```python
from build123d import *

# Parameters (mm, degrees)
STOCK_DGT_START                               = 23.8125
STOCK_DGT_INSIDE_SWERVE_STRUCTURE_SM_2_R      = 28.175
STOCK_DGT_INSIDE_SWERVE_STRUCTURE_SM_2_R_2    = 2.2479
STOCK_DGT_INSIDE_SWERVE_STRUCTURE_SMALL_DEPTH = 4.7625
FILLET1_R                                     = 1.905


# Read off the part's stored shape, not the designer's step: Stock-DGT inside swerve structure Small Bearing-1
with BuildPart() as part:
    # Stock-DGT inside swerve structure Sm 2 → Stock-DGT inside swerve structure Small Bearing-1 (new body)
    with BuildSketch(Plane(origin=(0, 0, 0), x_dir=(1, 0, 0), z_dir=(0, 1, 0)).offset(STOCK_DGT_START)):
        Circle(STOCK_DGT_INSIDE_SWERVE_STRUCTURE_SM_2_R)
        with Locations((-14.933176064, -16.8275)):
            Circle(STOCK_DGT_INSIDE_SWERVE_STRUCTURE_SM_2_R_2, mode=Mode.SUBTRACT)
        with Locations((14.933176064, -16.8275)):
            Circle(STOCK_DGT_INSIDE_SWERVE_STRUCTURE_SM_2_R_2, mode=Mode.SUBTRACT)
        with Locations((-14.933176064, 16.8275)):
            Circle(STOCK_DGT_INSIDE_SWERVE_STRUCTURE_SM_2_R_2, mode=Mode.SUBTRACT)
        with BuildLine():
            ThreePointArc((11.1125, 13.879508051), (12.572358569, 12.572358569), (13.879508051, 11.1125))
            Line((13.879508051, 11.1125), (22.394471276, 11.1125))
            ThreePointArc((22.394471276, 11.1125), (25, 0), (22.394471276, -11.1125))
            Line((22.394471276, -11.1125), (13.879508051, -11.1125))
            ThreePointArc((13.879508051, -11.1125), (12.572358569, -12.572358569), (11.1125, -13.879508051))
            Line((11.1125, -13.879508051), (11.1125, -19.116031394))
            Line((11.1125, -19.116031394), (-11.1125, -19.116031394))
            Line((-11.1125, -19.116031394), (-11.1125, -11.33701763))
            ThreePointArc((-11.1125, -11.33701763), (-15.875, 0), (-11.1125, 11.33701763))
            Line((-11.1125, 11.33701763), (-11.1125, 19.116031394))
            Line((-11.1125, 19.116031394), (11.1125, 19.116031394))
            Line((11.1125, 19.116031394), (11.1125, 13.879508051))
        make_face(mode=Mode.SUBTRACT)
        with Locations((14.933176064, 16.8275)):
            Circle(STOCK_DGT_INSIDE_SWERVE_STRUCTURE_SM_2_R_2, mode=Mode.SUBTRACT)
    extrude(amount=STOCK_DGT_INSIDE_SWERVE_STRUCTURE_SMALL_DEPTH)

    # Fillet1
    fillet1_edges = [part.edges().sort_by_distance(p)[0] for p in [
        (22.394471276, 26.19375, 11.1125),
        (22.394471276, 26.19375, -11.1125),
        (11.1125, 26.19375, 13.879508051),
        (11.1125, 26.19375, -13.879508051),
        (13.879508051, 26.19375, -11.1125),
        (13.879508051, 26.19375, 11.1125),
        (-11.1125, 26.19375, -11.33701763),
        (-11.1125, 26.19375, 11.33701763),
        (11.1125, 26.19375, -19.116031394),
        (-11.1125, 26.19375, 19.116031394),
        (11.1125, 26.19375, 19.116031394),
        (-11.1125, 26.19375, -19.116031394),
    ]]
    fillet(fillet1_edges, radius=FILLET1_R)


solid = part.part
```
Check sheet for the modelled part. Datum: model origin and axes. Units: mm. Round coordinates to 2 decimals unless told otherwise and drop trailing zeros. Loops run counter-clockwise (first coordinate to the right, second up) from the corner with the lowest first, then second, coordinate; pieces in that order, holes last. Notation, with made-up numbers: (-7, 47) -> (19, 47) arc R25 ccw to (19, 75) -> close; hole circle Ø1 at (-23, -37.75). An arc over 180 degrees is marked (long way). Answer in a Markdown table with one row per item.
Q1. Go/stop test with flat-tipped pins: P1, Ø1.4, axis at x = 18, y = 27, coming from the +Z side; P2, Ø4, axis at x = -14.93, z = 16.83, coming from the +Y side; P3, Ø2.5, axis at y = 27, z = -16, coming from the -X side; P4, Ø2, axis at y = 26.5, z = 16, coming from the -X side. Record where each tip stops, or that it passes through.
Data:
| item | result |
|---|---|
| P1 | stops at z = 22.24 |
| P2 | passes through |
| P3 | stops at x = -24.01 |
| P4 | stops at x = -23.85 |
Q2. Sectioned sample at A-A on x = 0. Enter the section's corners in (y, z) (1 decimal).
Data:
| item | result |
|---|---|
| outline | (23.8, -28.2) -> (28.6, -28.2) -> (28.6, -19.1) -> (23.8, -19.1) -> close; (23.8, 19.1) -> (28.6, 19.1) -> (28.6, 28.2) -> (23.8, 28.2) -> close |
Q3. Thickness scan on L1, parallel to Z at x = 0.5, y = 26.5; L2, parallel to Z at x = 14, y = 24.9; L3, parallel to X at y = 27.4, z = 17.5. Record the ranges inside material, lowest first.
Data:
| item | result |
|---|---|
| L1 | z = -28.17 to -19.12, 19.12 to 28.17 |
| L2 | z = -24.45 to -18.87, -14.78 to -11.27, 11.27 to 14.78, 18.87 to 24.45 |
| L3 | x = -22.08 to -17.08, -12.79 to -11.09, 11.09 to 12.79, 17.08 to 22.08 |
Q4. Sectioned sample at C-C on z = -18. Enter the section's corners in (x, y) (1 decimal).
Data:
| item | result |
|---|---|
| outline | (-21.7, 23.8) -> (-16.9, 23.8) -> (-16.9, 28.6) -> (-21.7, 28.6) -> close; (-13, 23.8) -> (-10.9, 23.8) -> (-10.9, 28.6) -> (-13, 28.6) -> close; (10.9, 23.8) -> (13, 23.8) -> (13, 28.6) -> (10.9, 28.6) -> close; (16.9, 23.8) -> (21.7, 23.8) -> (21.7, 28.6) -> (16.9, 28.6) -> close |
Q5. Sectioned sample at D-D on y = 26.2. Give the number of separate pieces and of enclosed holes in the cut face, then the cut area to 3 significant figures.
Data:
| item | result |
|---|---|
| separate pieces | 1 |
| enclosed holes | 5 |
| area | 1,210 mm^2 |
Q6. Sectioned sample at B-B on z = 0. Enter the section's corners in (x, y) (1 decimal).
Data:
| item | result |
|---|---|
| outline | (-28.2, 23.8) -> (-15.9, 23.8) -> (-15.9, 28.6) -> (-28.2, 28.6) -> close; (25, 23.8) -> (28.2, 23.8) -> (28.2, 28.6) -> (25, 28.6) -> close |
